Design review of the part built by this model. Coordinates are the model's own, in mm. A direction names the side the tool comes from. Coordinates: 2 decimals unless noted, no trailing zeros. Loops run counter-clockwise (first coordinate to the right, second up) from the corner with the lowest first, then second, coordinate; pieces in that order, holes last. Notation, with made-up numbers: M -33.5,-38.75 L -12.5,-38.75 A23 cw -12.5,-27.75 Z; hole C 46,18.25 d9. An arc over 180 degrees is marked long. One line per item, written item: value.
```python
from build123d import *

# Parameters (mm, degrees)
F1_DEPTH  = 76.2
F2_R      = 12.7
F3_DEPTH  = 76.201
F5_DEPTH  = 25.401
F6_R      = 38.1
F7_R      = 38.1
F8_R      = 15.875
F8_R_2    = 12.7
F9_DEPTH  = 6.35
F12_DEPTH = 12.7


with BuildPart() as f1:
    # F0 (on Front) → F1 (new body, symmetric)
    with BuildSketch(Plane.XZ):
        Polygon((-76.2, 0), (0, 0), (0, 152.4), (-25.4, 152.4), (-25.4, 25.4), (-76.2, 25.4), align=None)
    extrude(amount=F1_DEPTH, both=True)

    # F2 (on face) → F3 (cut, through all)
    with BuildSketch(Plane.YZ):
        with Locations((0, 114.3)):
            Circle(F2_R)
    extrude(amount=-F3_DEPTH, mode=Mode.SUBTRACT)

    # F4 (on face) → F5 (cut, through all)
    with BuildSketch(Plane.XY.offset(25.4)):
        with BuildLine():
            Line((-76.2, 12.7), (-76.2, 0))
            Line((-76.2, 0), (-76.2, -12.7))
            Line((-76.2, -12.7), (-63.5, -12.7))
            ThreePointArc((-63.5, -12.7), (-50.8, 0), (-63.5, 12.7))
            Line((-63.5, 12.7), (-76.2, 12.7))
        make_face()
    extrude(amount=-F5_DEPTH, mode=Mode.SUBTRACT)

    # F6
    f6_edges = [f1.edges().sort_by_distance(p)[0] for p in [
        (-12.7, -76.2, 152.4),
    ]]
    fillet(f6_edges, radius=F6_R)

    # F7
    f7_edges = [f1.edges().sort_by_distance(p)[0] for p in [
        (-12.7, 76.2, 152.4),
    ]]
    fillet(f7_edges, radius=F7_R)

    # F8 (on face) → F9 (cut)
    with BuildSketch(Plane(origin=(-25.4, 0, 0), x_dir=(0, -1, 0), z_dir=(-1, 0, 0))):
        with Locations((0, 114.3)):
            Circle(F8_R)
        with Locations((0, 114.3)):
            Circle(F8_R_2, mode=Mode.SUBTRACT)
    extrude(amount=-F9_DEPTH, mode=Mode.SUBTRACT)

    # F11 (on offset) → F12 (join)
    with BuildSketch(Plane.XZ.offset(44.45)):
        Polygon((-50.8, 25.4), (-25.4, 25.4), (-25.4, 114.3), align=None)
    extrude(amount=F12_DEPTH)


solid = f1.part
```
(1) We need section A-A on y = 0. State the section outline as (x, z) points (3 decimals).
Reply:
outline: M -50.8,0 L 0,0 L 0,101.6 L -19.05,101.6 L -19.05,98.425 L -25.4,98.425 L -25.4,25.4 L -50.8,25.4 Z; M -25.4,130.175 L -19.05,130.175 L -19.05,127 L 0,127 L 0,152.4 L -25.4,152.4 Z
(2) We need section D-D on x = -35.5. State the section outline as (y, z) points, then the cut area to 3 significant figures.
Reply:
outline: M -76.2,0 L 76.2,0 L 76.2,25.4 L -44.45,25.4 L -44.45,78.95 L -57.15,78.95 L -57.15,25.4 L -76.2,25.4 Z
area: 4,550 mm2
(3) Tool access review of faces 1 (the cylindrical face through (-9.39, -2.75, 101.9)), 2 (the flat face through (-70, -12.7, 13)), 3 (the flat face through (-19.05, 0.1, 127.3)): name each direction out of +Z, -Z, +X, -X, +Y, -Y from which nothing blocks a thin tool from reaching the whole face with its end or side.
Reply:
face 1: +X, -X
face 2: +Z, -Z, -X
face 3: -X
(4) Mouldability with a two-part tool opening along Y and no side actions: class faces 4 (the flat face through (-33, -57.15, 51)), 5 (the cylindrical face through (-12.88, 64.74, 141.54)), 6 (the cylindrical face through (-22.27, -8.53, 127.69)) as released by +Y, released by -Y, zero draft, split by the parting line, or undercut.
Reply:
face 4: released by -Y
face 5: released by +Y
face 6: undercut
(5) We need section C-C on z = 45. State the section outline as (x, y) points.
Reply:
outline: M -45.2,-57.15 L -25.4,-57.15 L -25.4,-76.2 L 0,-76.2 L 0,76.2 L -25.4,76.2 L -25.4,-44.45 L -45.2,-44.45 Z
(6) To check wall thickness, follow line 1 along Z through (x, y) = (-22.5, 0) (3 decimals); line 2 along Y through (x, z) = (-22, 114); line 3 along Z through (x, y) = (-11, 0). State the ranges of each line that lie inside material, in increasing order. Write a range as [from, to].
Reply:
line 1: z = [0, 98.425], [130.175, 152.4]
line 2: y = [-76.2, -15.87], [15.87, 76.2]
line 3: z = [0, 101.6], [127, 152.4]
(7) We need section B-B on x = -21.5. State the section outline as (y, z) points (3 decimals).
Reply:
outline: M -76.2,0 L 76.2,0 L 76.2,114.3 A38.1 ccw 38.1,152.4 L -38.1,152.4 A38.1 ccw -76.2,114.3 Z; hole C 0,114.3 d31.75
(8) Insertion check: pin 1 (1 mm diameter, centred on x = -66.5, y = -56, fed in from +Z); pin 2 (12.5 mm diameter, centred on x = -41.5, z = 56.5, fed in from +Y); pin 3 (16 mm diameter, centred on y = 7.5, z = 117.5, fed in from -X). Each pin has a flat end and moves straight along its axis. Give the tip position at first contact, or say it passes through.
Reply:
pin 1: stops at z = 25.4
pin 2: stops at y = -44.45
pin 3: stops at x = -25.4
